CAD build for the part. Positions are in the model's coordinates, mm. Coordinates: 2 decimals unless noted, no trailing zeros. Write each loop counter-clockwise with the first axis right and the second up, starting at its lowest first coordinate (ties: lowest second). Pieces come first, ordered by that corner, then holes. Notation, with made-up numbers: (16, 53) - (72, 53) arc R33 ccw to (72, 86) - close; hole circle Ø10 at (43, 0.5). An arc over 180 degrees is marked (long way). Answer in a Markdown table with one row per item. Add a question column.
Q1. Pin check, flat tips, straight feed: pin 1 (1.5 mm diameter, centred on y = -0.5, z = 5, fed in from +X); pin 2 (1.5 mm diameter, centred on y = 0, z = 5, fed in from -X); pin 3 (1 mm diameter, centred on y = -2, z = 6, fed in from -X). Stop position of each tip, or through.
Q2. Band-saw the part on C-C (z = 3.25). List the corners of the cut face in (x, y), and give its area (3 significant figures).
Q3. Band-saw the part on A-A (y = 0). List the corners of the cut face in (x, z).
Q4. Two-plate mould, pull along Y, no slides. Class faces 1 (the cylindrical face through (-2.947, 0.13, 3.944)), 2 (the flat face through (1, -3, 8)): +Y half, -Y half, draft (parallel to the pull), parting line (faces both ways), or undercut.
Q5. Drill centre lines: line 1 along Z through (x, y) = (-3.25, -1.5); line 2 along Z through (x, y) = (-1.25, -4); line 3 along X through (y, z) = (-2.5, 2.75). Where is each one in solid material? Low to high. Write a range as from..to.
```python
from build123d import *

# Parameters (mm, degrees)
CYLINDER003_R     = 4.5
CYLINDER003_DEPTH = 1
FILLET001_R       = 0.9
CYLINDER002_R     = 2.95
CYLINDER002_DEPTH = 8


with BuildPart() as fillet001:
    # Cylinder003 → Cylinder003 (new body)
    with BuildSketch(Plane.XY.offset(8)):
        Circle(CYLINDER003_R)
    extrude(amount=CYLINDER003_DEPTH)

    # Fillet001
    fillet001_edges = [fillet001.edges().sort_by_distance(p)[0] for p in [
        (-4.5, 0, 9),
    ]]
    fillet(fillet001_edges, radius=FILLET001_R)


with BuildPart() as fusion001:
    # Cylinder002 → Cylinder002 (new body)
    with BuildSketch(Plane.XY):
        Circle(CYLINDER002_R)
    extrude(amount=CYLINDER002_DEPTH)

    # Fusion001: union Fillet001
    add(fillet001.part)


solid = fusion001.part
```
Checked values:
| question | item | result |
|---|---|---|
| 1 | pin 1 | stops at x = 2.95 |
| 1 | pin 2 | stops at x = -2.95 |
| 1 | pin 3 | stops at x = -2.54 |
| 2 | outline | circle Ø5.9 at (0, 0) |
| 2 | area | 27.3 mm² |
| 3 | outline | (-4.5, 8) - (-2.95, 8) - (-2.95, 0) - (2.95, 0) - (2.95, 8) - (4.5, 8) - (4.5, 8.1) arc R0.9 ccw to (3.6, 9) - (-3.6, 9) arc R0.9 ccw to (-4.5, 8.1) - close |
| 4 | face 1 | parting line |
| 4 | face 2 | draft |
| 5 | line 1 | z = 8..9 |
| 5 | line 2 | z = 8..8.78 |
| 5 | line 3 | x = -1.57..1.57 |
